```python
from build123d import *

# Parameters (mm, degrees)
SKETCH1_W           = 7.6
SKETCH1_H           = 7
BOSS_EXTRUDE1_DEPTH = 1
SKETCH2_R           = 2
CUT_EXTRUDE1_DEPTH  = 6.262128847
FILLET1_R           = 0.2


with BuildPart() as part:
    # Sketch1 → Boss-Extrude1 (new body)
    with BuildSketch(Plane(origin=(0, 0, 0), x_dir=(1, 0, 0), z_dir=(0, 1, 0))):
        Rectangle(SKETCH1_W, SKETCH1_H)
    extrude(amount=BOSS_EXTRUDE1_DEPTH)

    # Sketch2 → Cut-Extrude1 (cut, through all)
    with BuildSketch(Plane(origin=(0, 1, 0), x_dir=(1, 0, 0), z_dir=(0, 1, 0))):
        with Locations(Location((0, 0, 0), (0, 0, 270))):
            Circle(SKETCH2_R)
    extrude(amount=-CUT_EXTRUDE1_DEPTH, mode=Mode.SUBTRACT)

    # Fillet1
    fillet1_edges = [part.edges().sort_by_distance(p)[0] for p in [
        (-3.8, 1, 0),
        (0, 1, -2),
        (0, 1, 3.5),
        (3.8, 1, 0),
        (3.8, 0.5, 3.5),
        (-3.8, 0.5, 3.5),
        (-3.8, 0.5, -3.5),
        (3.8, 0.5, -3.5),
        (0, 1, -3.5),
    ]]
    fillet(fillet1_edges, radius=FILLET1_R)


solid = part.part
```
Here's how the part is built. I have some questions about the finished solid (model axes, mm). Coordinates: 2 decimals unless noted, no trailing zeros. Loops run counter-clockwise (first coordinate to the right, second up) from the corner with the lowest first, then second, coordinate; pieces in that order, holes last. Notation, with made-up numbers: (9, 49.25) -> (39, 49.25) arc R4 ccw to (39, 55.25) -> close; hole circle Ø2 at (20.25, -34.5). An arc over 180 degrees is marked (long way). Return JSON: item names as keys, results as strings.
1) If we section it at B-B, the plane y = 0.3: Write out the boundary of the cut face in (x, z), then the cut area to 3 significant figures.
Results below:
{"outline": "(-3.8, -3.3) arc R0.2 ccw to (-3.6, -3.5) -> (3.6, -3.5) arc R0.2 ccw to (3.8, -3.3) -> (3.8, 3.3) arc R0.2 ccw to (3.6, 3.5) -> (-3.6, 3.5) arc R0.2 ccw to (-3.8, 3.3) -> close; hole circle Ø4 at (0, 0)", "area": "40.6 mm²"}
2) Thinking about a two-plate mould opening in X: for faces 1 (the face through (-2, 0, 2)), 2 (the face through (-1.952, 0.406, -0.434)), which applies, +X half, -X half, draft (parallel to the pull), parting line (faces both ways), or undercut?
Results below:
{"face 1": "draft", "face 2": "undercut"}
3) If we section it at A-A, the plane x = 0: Write out the boundary of the cut face in (y, z).
Results below:
{"outline": "(0, -3.5) -> (0.8, -3.5) arc R0.2 ccw to (1, -3.3) -> (1, -2.2) arc R0.2 ccw to (0.8, -2) -> (0, -2) -> close; (0, 2) -> (0.8, 2) arc R0.2 ccw to (1, 2.2) -> (1, 3.3) arc R0.2 ccw to (0.8, 3.5) -> (0, 3.5) -> close"}
4) If we section it at C-C, the plane z = 0: Write out the boundary of the cut face in (x, y).
Results below:
{"outline": "(-3.8, 0) -> (-2, 0) -> (-2, 0.8) arc R0.2 ccw to (-2.2, 1) -> (-3.6, 1) arc R0.2 ccw to (-3.8, 0.8) -> close; (2, 0) -> (3.8, 0) -> (3.8, 0.8) arc R0.2 ccw to (3.6, 1) -> (2.2, 1) arc R0.2 ccw to (2, 0.8) -> close"}
5) I need wall thicknesses on line 1 (X direction, y = 0.6, z = 0); line 2 (X direction, y = 0.15, z = 1.75); line 3 (Z direction, x = -0.5, y = 0.65). Which ranges of each line are inside material? Lowest first, please. Write a range as from..to.
Results below:
{"line 1": "-3.8..-2, 2..3.8", "line 2": "-3.8..-0.97, 0.97..3.8", "line 3": "-3.5..-1.94, 1.94..3.5"}
